from build123d import *

# Parameters (mm, degrees)
SKETCH1_W             = 152.4
SKETCH1_H             = 28.575
SKETCH1_R             = 1.5875
BOSS_EXTRUDE1_DEPTH   = 4.699
SKETCH2_R             = 13.97
CUT_EXTRUDE1_DEPTH    = 1.778
F_4_40_TAPPED_HOLE1_D = 2.2606


with BuildPart() as part:
    # Sketch1 → Boss-Extrude1 (new body)
    with BuildSketch(Plane(origin=(0, 0, 0), x_dir=(1, 0, 0), z_dir=(0, 1, 0))):
        with Locations((76.2, 14.2875)):
            Rectangle(SKETCH1_W, SKETCH1_H)
        with Locations(Location((19.05, 17.0434, 0), (0, 0, 270))):
            Circle(SKETCH1_R, mode=Mode.SUBTRACT)
        with Locations(Location((47.625, 17.0434, 0), (0, 0, 270))):
            Circle(SKETCH1_R, mode=Mode.SUBTRACT)
        with Locations(Location((76.2, 17.0434, 0), (0, 0, 270))):
            Circle(SKETCH1_R, mode=Mode.SUBTRACT)
        with Locations(Location((104.775, 17.0434, 0), (0, 0, 270))):
            Circle(SKETCH1_R, mode=Mode.SUBTRACT)
        with Locations(Location((133.35, 17.0434, 0), (0, 0, 270))):
            Circle(SKETCH1_R, mode=Mode.SUBTRACT)
    extrude(amount=BOSS_EXTRUDE1_DEPTH)

    # Sketch2 → Cut-Extrude1 (cut)
    with BuildSketch(Plane.XZ):
        with Locations((19.05, -17.0434)):
            Circle(SKETCH2_R)
        with Locations((47.625, -17.0434)):
            Circle(SKETCH2_R)
        with Locations((76.2, -17.0434)):
            Circle(SKETCH2_R)
        with Locations((104.775, -17.0434)):
            Circle(SKETCH2_R)
        with Locations((133.35, -17.0434)):
            Circle(SKETCH2_R)
    extrude(amount=-CUT_EXTRUDE1_DEPTH, mode=Mode.SUBTRACT)

    # #4-40 Tapped Hole1 (through all)
    with Locations(Plane(origin=(0, 4.699, 0), x_dir=(1, 0, 0), z_dir=(0, 1, 0))):
        with Locations((3.175, 25.4), (3.175, 3.175), (149.225, 3.175), (149.225, 25.4)):
            Hole(F_4_40_TAPPED_HOLE1_D / 2)


solid = part.part
CAD build for the part. Positions are in the model's coordinates, mm. A direction names the side the tool comes from. Give positions to 0.01 mm unless a question says otherwise; leave off trailing zeros. Write each loop counter-clockwise with the first axis right and the second up, starting at its lowest first coordinate (ties: lowest second). Pieces come first, ordered by that corner, then holes. Notation, with made-up numbers: M -34.5,-2 L 1.5,-2 A11 cw 1.5,17 Z; hole C 61,19.5 d7. An arc over 180 degrees is marked long. Put each result on its own line as item: value. Start each with the question number.
(1) Band-saw the part on D-D, the plane z = -21.75. Write the cut outline in (x, y).
(2) Probe L1, parallel to X at y = 3.8, z = -25.25; L2, parallel to X at y = 0.5, z = -16.5; L3, parallel to X at y = 3.25, z = -25.4. List the from-to ranges inside material, lowest first.
(3) Flat gauge pins, fed straight in: pin 1 Ø3.5 at (x, z) = (149.225, -3.175) entering from +Y; pin 2 Ø3 at (x, z) = (76.2, -17.04) entering from -Y; pin 3 Ø2 at (x, z) = (116.5, -19.5) entering from -Y. Where does each tip first touch, or does it go through?
(4) Band-saw the part on A-A, the plane x = 76.2. Write the cut outline in (y, z) (3 decimals), and give its area (3 significant figures).
(5) Band-saw the part on C-C, the plane x = 108.5. Write the cut outline in (y, z) (3 decimals).
(6) Which spindle directions (+Z, -Z, +X, -X, +Y, -Y) get a long thin tool onto all of the face, cutting with end or side? Do faces 1 (the face through (75, 3, -28.575)), 2 (the face through (130, 1.778, -16)). Say none if no direction does.
(7) Band-saw the part on B-B, the plane z = -6. Write the cut outline in (x, y).
(8) Mould opens along X. For faces 3 (the face through (152.4, 2, -14)), 4 (the face through (75, 2, 0)), 5 (the face through (134.924, 3.218, -17.25)) say: +X half, -X half, draft (parallel to the pull), parting line (faces both ways), or undercut.
Response values:
1. outline: M 0,0 L 5.9,0 L 5.9,1.78 L 32.2,1.78 L 32.2,0 L 34.47,0 L 34.47,1.78 L 60.78,1.78 L 60.78,0 L 63.05,0 L 63.05,1.78 L 89.35,1.78 L 89.35,0 L 91.62,0 L 91.62,1.78 L 117.93,1.78 L 117.93,0 L 120.2,0 L 120.2,1.78 L 146.5,1.78 L 146.5,0 L 152.4,0 L 152.4,4.7 L 0,4.7 Z
2. L1: x = 0 to 2.05, 4.3 to 148.1, 150.35 to 152.4
2. L2: x = 0 to 5.09, 33.01 to 33.67, 61.58 to 62.24, 90.16 to 90.82, 118.73 to 119.39, 147.31 to 152.4
2. L3: x = 0 to 2.04, 4.31 to 148.09, 150.36 to 152.4
3. pin 1: stops at y = 4.7
3. pin 2: passes through
3. pin 3: stops at y = 1.78
4. outline: M 0,-3.073 L 1.778,-3.073 L 1.778,-15.456 L 4.699,-15.456 L 4.699,0 L 0,0 Z; M 1.778,-28.575 L 4.699,-28.575 L 4.699,-18.631 L 1.778,-18.631 Z
4. area: 79.7 mm2
5. outline: M 0,-3.579 L 1.778,-3.579 L 1.778,-28.575 L 4.699,-28.575 L 4.699,0 L 0,0 Z
6. face 1: -Z, +X, -X, +Y, -Y
6. face 2: -Y
7. outline: M 0,0 L 10.49,0 L 10.49,1.78 L 27.61,1.78 L 27.61,0 L 39.07,0 L 39.07,1.78 L 56.18,1.78 L 56.18,0 L 67.64,0 L 67.64,1.78 L 84.76,1.78 L 84.76,0 L 96.22,0 L 96.22,1.78 L 113.33,1.78 L 113.33,0 L 124.79,0 L 124.79,1.78 L 141.91,1.78 L 141.91,0 L 152.4,0 L 152.4,4.7 L 0,4.7 Z
8. face 3: +X half
8. face 4: draft
8. face 5: undercut
